Verification items for the finished model (mm, model axes). A direction names the side the tool comes from. Round coordinates to 2 decimals unless told otherwise and drop trailing zeros. Write each loop counter-clockwise with the first axis right and the second up, starting at its lowest first coordinate (ties: lowest second). Pieces come first, ordered by that corner, then holes. Notation, with made-up numbers: M -20.75,-20 L 33.25,-20 A12 ccw 33.25,-15 Z; hole C 45,59 d5. An arc over 180 degrees is marked long. One line per item, written item: value. Start each with the question number.
Item 1: Section check C-C, the plane x = 0. Record the cut outline in (y, z) (1 decimal).
Item 2: Tool access check on faces 5 (the face through (12.7, 0, -37)), 6 (the face through (18.497, -9.356, -53.842)), 7 (the face through (25.4, 0, -31)), 8 (the face through (6, -6, -3.81)). Record the directions out of +Z, -Z, +X, -X, +Y, -Y that give a thin tool (end or side, any length) a straight path to the whole face; none if there is none.
Item 3: Section check B-B, the plane y = 0. Record the cut outline in (x, z) (1 decimal), then the cut area to 3 significant figures.
Item 4: Section check A-A, the plane z = -22.5. Record the cut outline in (x, y).
Item 5: Thickness scan on probe 1 along Y at (x, z) = (19, -59); probe 2 along X at (y, z) = (-6, -24.5); probe 3 along Z at (x, y) = (-5.5, -14) (3 decimals). Record the ranges inside material, lowest first. Write a range as from..to.
Item 6: Gauge pin test, flat ends, axial feed: pin 1 (5 mm diameter, centred on x = 19.05, y = -11.11, fed in from -Z); pin 2 (3 mm diameter, centred on x = 19.05, y = 11.11, fed in from +Z); pin 3 (1 mm diameter, centred on x = 8.5, z = -12, fed in from -Y); pin 4 (3.5 mm diameter, centred on x = 19.05, y = -11.11, fed in from +Z). Record the tip position at first contact, or that the pin passes through.
Item 7: Draft check along X on faces 1 (the face through (-20.603, 12.102, -53.842)), 2 (the face through (-17, -17.462, -31)), 3 (the face through (-25.4, 0, -31)), 4 (the face through (18.497, 9.356, -9.658)). Enter one of: +X half, -X half, draft (parallel to the pull), parting line (faces both ways), or undercut.
Item 8: Section check D-D, the plane x = -9. Record the cut outline in (y, z) (1 decimal).
Autodesk Inventor part; units mm, degrees
ref_plane "YZ Plane" through (0, 0, 0) normal (1, 0, 0) x (0, 1, 0)
ref_plane "XZ Plane" through (0, 0, 0) normal (0, 1, 0) x (-1, 0, 0)
ref_plane "XY Plane" through (0, 0, 0) normal (0, 0, 1) x (1, 0, 0)
sketch "Sketch1" plane through (0, 0, 0) normal (0, 0, 1) x (1, 0, 0)
  line L0 (-35.56, 0) -> (35.56, 0)
  line L1 (0, -24.4475) -> (0, 24.4475)
  circle A0 centre (0, 0) radius 14.2875 construction
  line L2 (-25.4, 17.4625) -> (25.4, 17.4625)
  line L3 (25.4, 17.4625) -> (25.4, -17.4625)
  line L4 (25.4, -17.4625) -> (-25.4, -17.4625)
  line L5 (-25.4, -17.4625) -> (-25.4, 17.4625)
  circle A1 centre (0, 0) radius 7.9375
  point P0 (0, 17.4625)
  point P1 (25.4, 0)
  dimension "d1" = 28.575
  dimension "d2" = 34.925
  dimension "d3" = 50.8
  dimension "d4" = 15.875
extrude "Extrusion1" add sketch "Sketch1" against normal blind 63.5 contours L5 L2 L1 A1 L0 | L0 A1 L1 L4 L5 | L1 L2 L3 L0 A1 | A1 L0 L3 L4 L1
sketch "Sketch2" plane through (0, 0, -63.5) normal (0, 0, -1) x (-1, 0, 0)
  circle A0 centre (0, 0) radius 7.9375
  line L0 (-25.4, 17.4625) -> (25.4, 17.4625)
  line L1 (25.4, -17.4625) -> (-25.4, -17.4625)
  line L2 (-12.7, 17.4625) -> (12.7, 17.4625)
  line L3 (12.7, 17.4625) -> (12.7, -17.4625)
  line L4 (12.7, -17.4625) -> (-12.7, -17.4625)
  line L5 (-12.7, -17.4625) -> (-12.7, 17.4625)
  point P0 (0, 17.4625)
  point P1 (0, 17.4625)
  dimension "d7" = 25.4
extrude "Extrusion2" cut sketch "Sketch2" against normal blind 53.975
sketch "Sketch3" plane through (0, 0, 0) normal (0, 0, 1) x (1, 0, 0)
  circle A0 centre (0, 0) radius 7.9375
  circle A1 centre (0, 0) radius 14.3256
  dimension "d10" = 28.6512
extrude "Extrusion3" cut sketch "Sketch3" against normal blind 3.81
sketch "Sketch5" plane through (0, 0, 0) normal (0, 0, 1) x (1, 0, 0)
  line L0 (-25.4, 17.4625) -> (25.4, 17.4625)
  line L1 (-25.4, -17.4625) -> (-25.4, 17.4625)
  line L2 (-35.56, 0) -> (35.56, 0)
  line L3 (0, -24.4475) -> (0, 24.4475)
  point P0 (-19.05, 11.1125)
  point P1 (19.05, 11.1125)
  point P2 (-19.05, -11.1125)
  point P3 (19.05, -11.1125)
  dimension "d13" = 6.35
  dimension "d14" = 6.35
hole "Hole1" at (-19.05, 11.1125, 0) at (19.05, 11.1125, 0) at (-19.05, -11.1125, 0) at (19.05, -11.1125, 0) direction (0, 0, -1) diameter 3.683 depth 19.05 tip angle 118
sketch "Sketch6" plane through (0, 0, -63.5) normal (0, 0, -1) x (-1, 0, 0)
  line L0 (12.7, 17.4625) -> (25.4, 17.4625)
  line L1 (35.56, 0) -> (-35.56, 0)
  line L2 (0, -24.4475) -> (0, 24.4475)
  point P0 (0, 0)
  point P1 (19.05, 11.1125)
  point P2 (19.05, 17.4625)
  point P3 (19.05, -11.1125)
  dimension "d22" = 6.35
hole "Hole2" at (-19.05, 11.1125, -63.5) at (-19.05, -11.1125, -63.5) direction (0, 0, 1) diameter 3.683 depth 19.05 tip angle 118
mirror "Mirror1" about plane through (0, 0, 0) normal (1, 0, 0) of "Hole2"
properties part number "mount pillow block inner"
Response values:
1. outline: M -17.5,-9.5 L -7.9,-9.5 L -7.9,-3.8 L -14.3,-3.8 L -14.3,0 L -17.5,0 Z; M 7.9,-9.5 L 17.5,-9.5 L 17.5,0 L 14.3,0 L 14.3,-3.8 L 7.9,-3.8 Z
2. face 5: -Z, +Y, -Y
2. face 6: -Z
2. face 7: +Z, -Z, +X, +Y, -Y
2. face 8: +Z
3. outline: M -25.4,-63.5 L -12.7,-63.5 L -12.7,-9.5 L -7.9,-9.5 L -7.9,-3.8 L -14.3,-3.8 L -14.3,0 L -25.4,0 Z; M 7.9,-9.5 L 12.7,-9.5 L 12.7,-63.5 L 25.4,-63.5 L 25.4,0 L 14.3,0 L 14.3,-3.8 L 7.9,-3.8 Z
3. area: 1,650 mm2
4. outline: M -25.4,-17.46 L -12.7,-17.46 L -12.7,17.46 L -25.4,17.46 Z; M 12.7,-17.46 L 25.4,-17.46 L 25.4,17.46 L 12.7,17.46 Z
5. probe 1: y = -17.46..-12.95, -9.27..9.27, 12.95..17.46
5. probe 2: x = -25.4..-12.7, 12.7..25.4
5. probe 3: z = -9.525..0
6. pin 1: stops at z = -63.5
6. pin 2: stops at z = -19.25
6. pin 3: passes through
6. pin 4: stops at z = -19.1
7. face 1: undercut
7. face 2: draft
7. face 3: -X half
7. face 4: undercut
8. outline: M -17.5,-9.5 L 17.5,-9.5 L 17.5,0 L 11.1,0 L 11.1,-3.8 L -11.1,-3.8 L -11.1,0 L -17.5,0 Z
